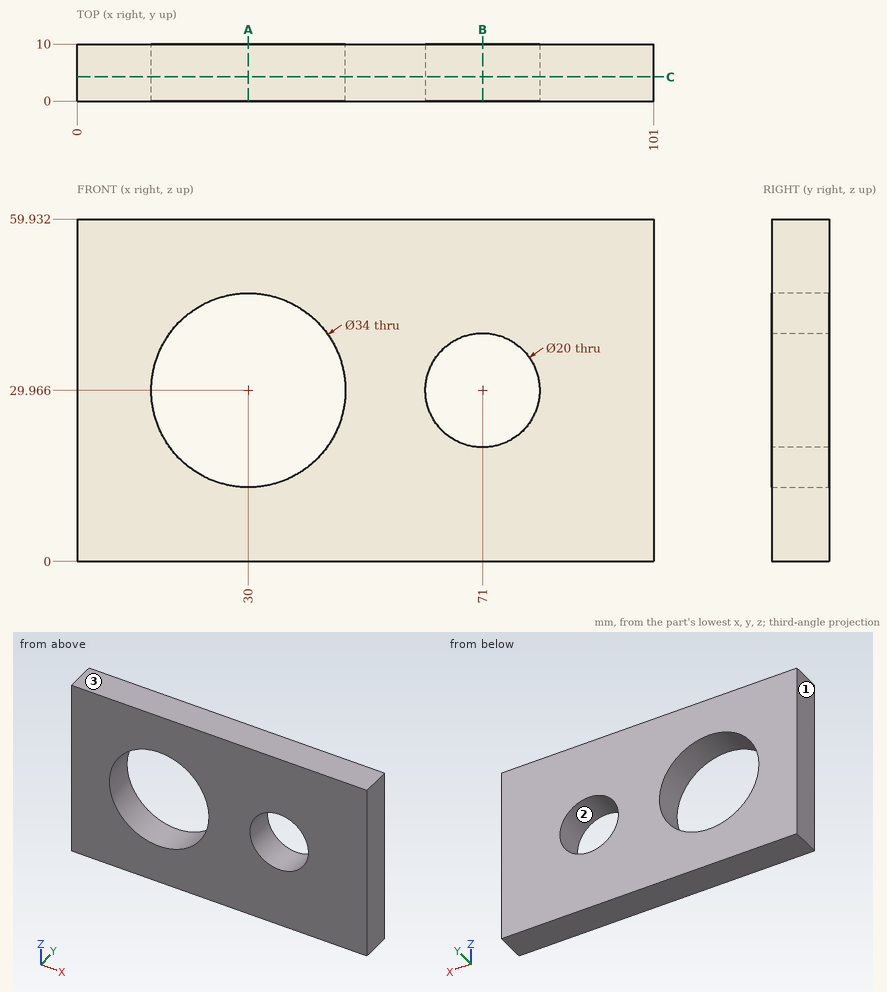
Geometry: see drawing. Coordinates: mm, zero at the bounding-box minimum. Round coordinates to 2 decimals unless told otherwise and drop trailing zeros. Order: outer loops, then holes, each group sorted by start corner. A loop starts at its lowest first (then second) coordinate and runs counter-clockwise, first axis right, second up. Notation, with made-up numbers: (-17, 34.5) - (14, 34.5) arc R18 cw to (14, 66.5) - close; hole circle Ø4 at (-6, -33.5). An arc over 180 degrees is marked (long way). Use a Markdown table: item, result. Add a question column.
1. Section query B-B (x = 71). Return the cut outline in (y, z).
2. Mould query, pull axis X, two halves, no side actions, for the marked faces 1, 2 and 3. Classes: +X half, -X half, draft (parallel to the pull), parting line (faces both ways), or undercut.
3. Line query: probe 1 along X at (y, z) = (3.5, 35); probe 2 along X at (y, z) = (8.75, 32); probe 3 along X at (y, z) = (2.25, 42.5) (1 decimal). Output: solid intervals per line, ascending.
4. Section query A-A (x = 30). Return the cut outline in (y, z), then the cut area to 3 significant figures.
5. Section query C-C (y = 4.25). Return the cut outline in (x, z), then the cut area to 3 significant figures.
Derived:
| question | item | result |
|---|---|---|
| 1 | outline | (0, 0) - (10, 0) - (10, 19.97) - (0, 19.97) - close; (0, 39.97) - (10, 39.97) - (10, 59.93) - (0, 59.93) - close |
| 2 | face 1 | -X half |
| 2 | face 2 | undercut |
| 2 | face 3 | draft |
| 3 | probe 1 | 0 to 13.76, 46.24 to 62.36, 79.64 to 101 |
| 3 | probe 2 | 0 to 13.12, 46.88 to 61.21, 80.79 to 101 |
| 3 | probe 3 | 0 to 18.5, 41.5 to 101 |
| 4 | outline | (0, 0) - (10, 0) - (10, 12.97) - (0, 12.97) - close; (0, 46.97) - (10, 46.97) - (10, 59.93) - (0, 59.93) - close |
| 4 | area | 259 mm2 |
| 5 | outline | (0, 0) - (101, 0) - (101, 59.93) - (0, 59.93) - close; hole circle Ø34 at (30, 29.97); hole circle Ø20 at (71, 29.97) |
| 5 | area | 4,830 mm2 |
